Geometry check sheet. Reference: drawing and pictorial views, mm from the part's lowest x, y, z. A direction names the side the tool comes from. Round coordinates to 2 decimals unless told otherwise and drop trailing zeros. Write each loop counter-clockwise with the first axis right and the second up, starting at its lowest first coordinate (ties: lowest second). Pieces come first, ordered by that corner, then holes. Notation, with made-up numbers: (-39.75, -39.5) -> (-35.75, -39.5) arc R28 ccw to (-35.75, -5.5) -> close; hole circle Ø11 at (55, 53.25). An arc over 180 degrees is marked (long way). Answer as a JSON object with one key per item and string values. Group by question number.
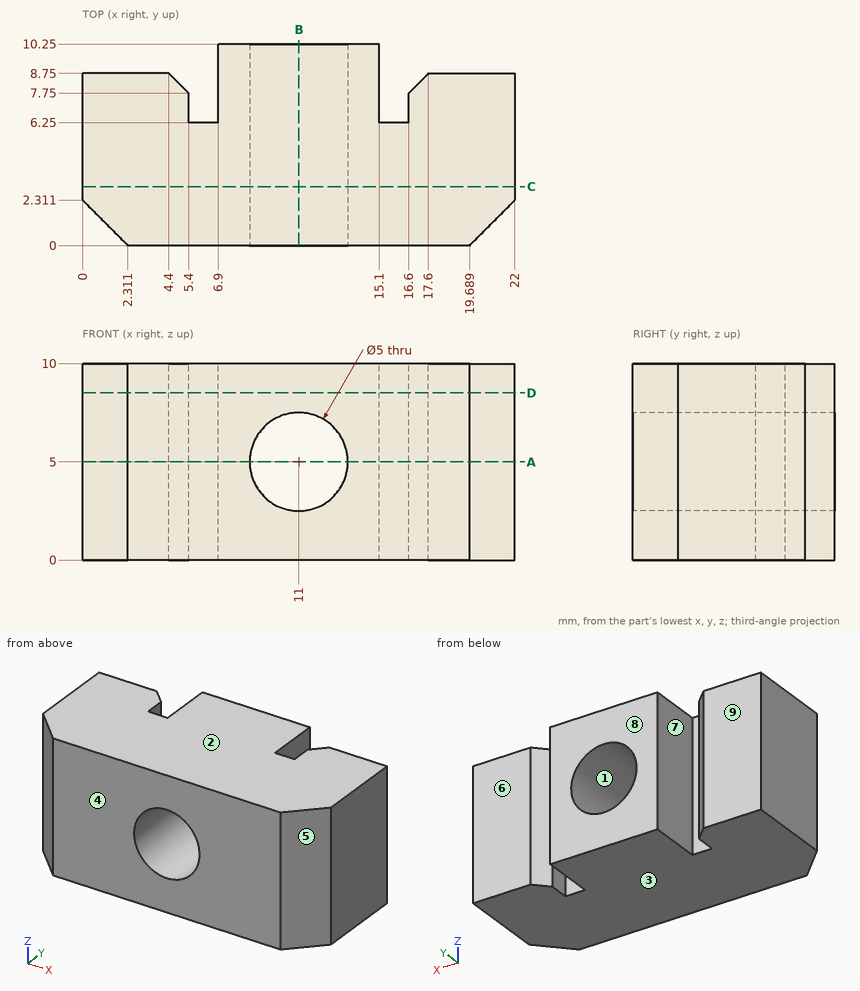
(1) Access from +Z, -Z, +X, -X, +Y, -Y to the whole of each face (thin tool, end or side, straight path). Record for the marked faces 5, 6, 7, 8 and 9.
(2) Section check D-D on z = 8.5. Record the cut outline in (x, y), then the cut area to 3 significant figures.
(3) Release check for a two-part mould opening along Z. For the marked faces 1, 2, 3 and 4 record: pulls with the +Z half, pulls with the -Z half, needs draft (parallel to the pull), parting line crosses it, or undercut.
(4) Section check C-C on y = 3. Record the cut outline in (x, z), then the cut area to 3 significant figures.
(5) Section check A-A on z = 5. Record the cut outline in (x, y).
(6) Go/stop test with a flat-tipped pin: pin 1 Ø5 at (x, z) = (3, 6.5) entering from +Y. Record where the tip stops, or that it passes through.
(7) Section check B-B on x = 11. Record the cut outline in (y, z).
(8) Scan lines: line 1 along X through (y, z) = (3.5, 5); line 2 along Z through (x, y) = (11, 5.25); line 3 along X through (y, z) = (8.25, 5). Record each from-to range of solid material in increasing order.
Data:
{
 "1": {"face 5": "+Z, -Z, +X, -Y", "face 6": "+Z, -Z, +X, +Y", "face 7": "+Z, -Z, +Y", "face 8": "+Z, -Z, +X, -X, +Y", "face 9": "+Z, -Z, -X, +Y"},
 "2": {"outline": "(0, 2.31) -> (2.31, 0) -> (19.69, 0) -> (22, 2.31) -> (22, 8.75) -> (17.6, 8.75) -> (16.6, 7.75) -> (16.6, 6.25) -> (15.1, 6.25) -> (15.1, 10.25) -> (6.9, 10.25) -> (6.9, 6.25) -> (5.4, 6.25) -> (5.4, 7.75) -> (4.4, 8.75) -> (0, 8.75) -> close", "area": "191 mm²"},
 "3": {"face 1": "undercut", "face 2": "pulls with the +Z half", "face 3": "pulls with the -Z half", "face 4": "needs draft"},
 "4": {"outline": "(0, 0) -> (22, 0) -> (22, 10) -> (0, 10) -> close; hole circle Ø5 at (11, 5)", "area": "200 mm²"},
 "5": {"outline": "(0, 2.31) -> (2.31, 0) -> (8.5, 0) -> (8.5, 10.25) -> (6.9, 10.25) -> (6.9, 6.25) -> (5.4, 6.25) -> (5.4, 7.75) -> (4.4, 8.75) -> (0, 8.75) -> close; (13.5, 0) -> (19.69, 0) -> (22, 2.31) -> (22, 8.75) -> (17.6, 8.75) -> (16.6, 7.75) -> (16.6, 6.25) -> (15.1, 6.25) -> (15.1, 10.25) -> (13.5, 10.25) -> close"},
 "6": {"pin 1": "stops at y = 8.75"},
 "7": {"outline": "(0, 0) -> (10.25, 0) -> (10.25, 2.5) -> (0, 2.5) -> close; (0, 7.5) -> (10.25, 7.5) -> (10.25, 10) -> (0, 10) -> close"},
 "8": {"line 1": "x = 0 to 8.5, 13.5 to 22", "line 2": "z = 0 to 2.5, 7.5 to 10", "line 3": "x = 0 to 4.9, 6.9 to 8.5, 13.5 to 15.1, 17.1 to 22"}
}
